Verification items for the finished model (mm, model axes). A direction names the side the tool comes from. Round coordinates to 2 decimals unless told otherwise and drop trailing zeros. Loops run counter-clockwise (first coordinate to the right, second up) from the corner with the lowest first, then second, coordinate; pieces in that order, holes last. Notation, with made-up numbers: M -38.5,-15.75 L -29.5,-15.75 A16 cw -29.5,2.25 Z; hole C 25,-22 d10. An arc over 180 degrees is marked long. Answer as CSV lines item,"result".
```python
from build123d import *

# Parameters (mm, degrees)
F1_DEPTH = 25.4
F2_R     = 4.7625
F3_DEPTH = 25.4


with BuildPart() as f1:
    # F0 (on Right) → F1 (new body, symmetric)
    with BuildSketch(Plane.YZ):
        Polygon((330.2, 9.525), (0, 9.525), (0, 0), (-29.345384, 0), (-33.290768, -9.525), (381, -9.525), (381, 0), (330.2, 0), align=None)
    extrude(amount=F1_DEPTH, both=True)

    # F2 (on Top) → F3 (cut)
    with BuildSketch(Plane.XY):
        with Locations((0, -9.525)):
            Circle(F2_R)
        with Locations((0, 371.475)):
            Circle(F2_R)
    extrude(amount=-F3_DEPTH, mode=Mode.SUBTRACT)


solid = f1.part
```
1) Draft check along Y on faces 1 (the flat face through (0, 356, 0)), 2 (the cylindrical face through (-1.032, 366.826, -4.696)), 3 (the flat face through (0, 330.2, 5)). Enter one of: +Y half, -Y half, draft (parallel to the pull), parting line (faces both ways), or undercut.
Here are the results:
face 1,"draft"
face 2,"undercut"
face 3,"+Y half"
2) Material ranges on probe 1 along Y at (x, z) = (0, -3); probe 2 along Y at (x, z) = (0, -5.25); probe 3 along Y at (x, z) = (8, 5.25), recorded low to high.
Here are the results:
probe 1,"y = -30.59 to -14.29, -4.76 to 366.71, 376.24 to 381"
probe 2,"y = -31.52 to -14.29, -4.76 to 366.71, 376.24 to 381"
probe 3,"y = 0 to 330.2"
3) Section check A-A (x = 0). Record the cut outline in (y, z) (1 decimal).
Here are the results:
outline,"M -33.3,-9.5 L -14.3,-9.5 L -14.3,0 L -29.3,0 Z; M -4.8,-9.5 L 366.7,-9.5 L 366.7,0 L 330.2,0 L 330.2,9.5 L 0,9.5 L 0,0 L -4.8,0 Z; M 376.2,-9.5 L 381,-9.5 L 381,0 L 376.2,0 Z"
4) Section check C-C (z = 4.75). Record the cut outline in (x, y), plus the area to 3 significant figures.
Here are the results:
outline,"M -25.4,0 L 25.4,0 L 25.4,330.2 L -25.4,330.2 Z"
area,"16,800 mm^2"
5) Set-up check for faces 4 (the flat face through (0, 0, 5)), 5 (the cylindrical face through (-0.6, -4.8, -4.7)): record each of +Z, -Z, +X, -X, +Y, -Y from which the full face is reachable in a straight line by a thin tool's end or side.
Here are the results:
face 4,"+Z, +X, -X, -Y"
face 5,"+Z, -Z"
6) Section check B-B (y = 336.5). Record the cut outline in (x, z) (3 decimals), plus the area to 3 significant figures.
Here are the results:
outline,"M -25.4,-9.525 L 25.4,-9.525 L 25.4,0 L -25.4,0 Z"
area,"484 mm^2"
7) Go/stop test with flat-tipped pins: pin 1 (5 mm diameter, centred on x = 6, z = 5.5, fed in from -Y); pin 2 (9 mm diameter, centred on x = -7, y = -7.5, fed in from +Z); pin 3 (5 mm diameter, centred on x = -9, z = 6.5, fed in from +Y); pin 4 (12.5 mm diameter, centred on x = 0, y = -9.525, fed in from -Z) (3 decimals). Record where each tip stops, or that it passes through.
Here are the results:
pin 1,"stops at y = 0"
pin 2,"stops at z = 0"
pin 3,"stops at y = 330.2"
pin 4,"stops at z = -9.525"
